Work out the finished part from the listing and answer in its coordinate system (mm). A direction names the side the tool comes from. Round coordinates to 2 decimals unless told otherwise and drop trailing zeros. Write each loop counter-clockwise with the first axis right and the second up, starting at its lowest first coordinate (ties: lowest second). Pieces come first, ordered by that corner, then holes. Notation, with made-up numbers: (17.5, 66.5) -> (74.5, 66.5) arc R10 cw to (74.5, 82.5) -> close; hole circle Ø11 at (17.25, 30.5). An arc over 180 degrees is marked (long way). One line per item, written item: value.
```python
from build123d import *

# Parameters (mm, degrees)
BOSS_EXTRUDE1_DEPTH  = 9.5
BOSS_EXTRUDE2_DEPTH  = 22
BOSS_EXTRUDE3_DEPTH  = 7.9
SKETCH5_R            = 11
SKETCH5_R_2          = 5
BOSS_EXTRUDE4_DEPTH  = 2
CUT_EXTRUDE1_START   = -3
SKETCH6_R            = 5
CUT_EXTRUDE1_DEPTH   = 3
SKETCH7_R            = 2.5
BOSS_EXTRUDE5_DEPTH  = 5
SKETCH8_R            = 2.5
BOSS_EXTRUDE6_DEPTH  = 22
CUT_EXTRUDE2_DEPTH   = 17
SKETCH11_W           = 3.2
SKETCH11_H           = 16
BOSS_EXTRUDE8_DEPTH  = 3.9
BOSS_EXTRUDE9_DEPTH  = 5.6
SKETCH13_W           = 0.930512921
SKETCH13_H           = 15
BOSS_EXTRUDE10_DEPTH = 3.9
SKETCH14_W           = 0.930512921
SKETCH14_H           = 15
BOSS_EXTRUDE11_DEPTH = 0.1
BOSS_EXTRUDE12_DEPTH = 5
SKETCH16_R           = 0.25
BOSS_EXTRUDE13_DEPTH = 5
SKETCH17_R           = 1.5
CUT_EXTRUDE3_DEPTH   = 5.5
SKETCH18_R           = 3.25
CUT_EXTRUDE4_DEPTH   = 3
CUT_EXTRUDE5_START   = -4
SKETCH20_R           = 1.5
CUT_EXTRUDE5_DEPTH   = 4
SKETCH21_R           = 4.5
CUT_EXTRUDE6_DEPTH   = 4


with BuildPart() as part:
    # Sketch1 → Boss-Extrude1 (new body)
    with BuildSketch(Plane.XY):
        Polygon((-17, 21), (-21, 17), (-21, -17), (-17, -21), (17, -21), (21, -17), (21, 17), (17, 21), align=None)
    extrude(amount=BOSS_EXTRUDE1_DEPTH)

    # Sketch2 → Boss-Extrude2 (add)
    with BuildSketch(Plane.XY.offset(9.5)):
        Polygon((14, 21.15), (21.15, 14), (21.15, -14), (14, -21.15), (-14, -21.15), (-21.15, -14), (-21.15, 14), (-14, 21.15), align=None)
    extrude(amount=BOSS_EXTRUDE2_DEPTH)

    # Sketch3 → Boss-Extrude3 (add)
    with BuildSketch(Plane.XY.offset(31.5)):
        Polygon((-17, 21), (17, 21), (21, 17), (21, -17), (17, -21), (-17, -21), (-21, -17), (-21, 17), align=None)
    extrude(amount=BOSS_EXTRUDE3_DEPTH)

    # Sketch5 → Boss-Extrude4 (add)
    with BuildSketch(Plane.XY.offset(39.4)):
        with Locations(Location((0, 0, 0), (0, 0, 180))):
            Circle(SKETCH5_R)
        Circle(SKETCH5_R_2, mode=Mode.SUBTRACT)
    extrude(amount=BOSS_EXTRUDE4_DEPTH)

    # Sketch6 → Cut-Extrude1 (cut)
    with BuildSketch(Plane.XY.offset(39.4).offset(CUT_EXTRUDE1_START)):
        Circle(SKETCH6_R)
    extrude(amount=CUT_EXTRUDE1_DEPTH, mode=Mode.SUBTRACT)

    # Sketch7 → Boss-Extrude5 (add)
    with BuildSketch(Plane.XY.offset(36.4)):
        with Locations(Location((0, 0, 0), (0, 0, 180))):
            Circle(SKETCH7_R)
    extrude(amount=BOSS_EXTRUDE5_DEPTH)

    # Sketch8 → Boss-Extrude6 (add)
    with BuildSketch(Plane.XY.offset(41.4)):
        with Locations(Location((0, 0, 0), (0, 0, 180))):
            Circle(SKETCH8_R)
    extrude(amount=BOSS_EXTRUDE6_DEPTH)

    # Sketch9 → Cut-Extrude2 (cut)
    with BuildSketch(Plane.XY.offset(63.4)):
        Polygon((-2.316645086, 2.1), (3.697939095, 2.1), (-0.123554347, 3.991048302), align=None)
    extrude(amount=-CUT_EXTRUDE2_DEPTH, mode=Mode.SUBTRACT)

    # Sketch11 → Boss-Extrude8 (add)
    with BuildSketch(Plane(origin=(21, 0, 0), x_dir=(0, 0, -1), z_dir=(1, 0, 0))):
        with Locations((-1.645589959, 0)):
            Rectangle(SKETCH11_W, SKETCH11_H)
    extrude(amount=BOSS_EXTRUDE8_DEPTH)

    # Sketch12 → Boss-Extrude9 (add)
    with BuildSketch(Plane(origin=(21, 0, 0), x_dir=(0, 0, -1), z_dir=(1, 0, 0))):
        Polygon((-9.5, 7.2), (-4.97610288, 7.2), (-4.97610288, -7.2), (-9.5, -7.2), (-9.5, -8), (-4.17610288, -8), (-4.17610288, -7.2), (-4.17610288, 7.2), (-4.17610288, 8), (-9.5, 8), align=None)
    extrude(amount=BOSS_EXTRUDE9_DEPTH)

    # Sketch13 → Boss-Extrude10 (add)
    with BuildSketch(Plane(origin=(21, 0, 0), x_dir=(0, 0, -1), z_dir=(1, 0, 0))):
        with Locations((-3.71084642, 0)):
            Rectangle(SKETCH13_W, SKETCH13_H)
    extrude(amount=BOSS_EXTRUDE10_DEPTH)

    # Sketch14 → Boss-Extrude11 (add)
    with BuildSketch(Plane(origin=(24.9, 0, 0), x_dir=(0, 0, -1), z_dir=(1, 0, 0))):
        with Locations((-3.71084642, 0)):
            Rectangle(SKETCH14_W, SKETCH14_H)
    extrude(amount=BOSS_EXTRUDE11_DEPTH)

    # Sketch15 → Boss-Extrude12 (add)
    with BuildSketch(Plane(origin=(21, 0, 0), x_dir=(0, 0, -1), z_dir=(1, 0, 0))):
        Polygon((-5.97610288, 6.2), (-9, 6.2), (-9, 4), (-9.5, 4), (-9.5, 6.7), (-9, 6.7), (-5.47610288, 6.7), (-5.47610288, -6.7), (-9, -6.7), (-9.5, -6.7), (-9.5, -4), (-9, -4), (-9, -6.2), (-5.97610288, -6.2), align=None)
    extrude(amount=BOSS_EXTRUDE12_DEPTH)

    # Sketch16 → Boss-Extrude13 (add)
    with BuildSketch(Plane(origin=(21, 0, 0), x_dir=(0, 0, -1), z_dir=(1, 0, 0))):
        with Locations(Location((-7.48805144, 5, 0), (0, 0, 270))):
            Circle(SKETCH16_R)
        with Locations(Location((-7.48805144, 3, 0), (0, 0, 270))):
            Circle(SKETCH16_R)
        with Locations(Location((-7.48805144, 1, 0), (0, 0, 270))):
            Circle(SKETCH16_R)
        with Locations(Location((-7.48805144, -1, 0), (0, 0, 270))):
            Circle(SKETCH16_R)
        with Locations(Location((-7.48805144, -3, 0), (0, 0, 270))):
            Circle(SKETCH16_R)
        with Locations(Location((-7.48805144, -5, 0), (0, 0, 270))):
            Circle(SKETCH16_R)
    extrude(amount=BOSS_EXTRUDE13_DEPTH)

    # Sketch17 → Cut-Extrude3 (cut)
    with BuildSketch(Plane.XY.offset(39.4)):
        with Locations((-15.5, 15.5)):
            Circle(SKETCH17_R)
        with Locations((15.5, 15.5)):
            Circle(SKETCH17_R)
        with Locations((15.5, -15.5)):
            Circle(SKETCH17_R)
        with Locations((-15.5, -15.5)):
            Circle(SKETCH17_R)
    extrude(amount=-CUT_EXTRUDE3_DEPTH, mode=Mode.SUBTRACT)

    # Sketch18 → Cut-Extrude4 (cut)
    with BuildSketch(Plane(origin=(0, 0, 0), x_dir=(-1, 0, 0), z_dir=(0, 0, -1))):
        with Locations((-15.5, 15.5)):
            Circle(SKETCH18_R)
        with Locations((15.5, 15.5)):
            Circle(SKETCH18_R)
        with Locations((15.5, -15.5)):
            Circle(SKETCH18_R)
        with Locations((-15.5, -15.5)):
            Circle(SKETCH18_R)
    extrude(amount=-CUT_EXTRUDE4_DEPTH, mode=Mode.SUBTRACT)

    # Sketch20 → Cut-Extrude5 (cut)
    with BuildSketch(Plane(origin=(0, 0, 3), x_dir=(-1, 0, 0), z_dir=(0, 0, -1)).offset(CUT_EXTRUDE5_START)):
        with Locations(Location((-15.5, 15.5, 0), (0, 0, 180))):
            Circle(SKETCH20_R)
        with Locations(Location((15.5, 15.5, 0), (0, 0, 180))):
            Circle(SKETCH20_R)
        with Locations(Location((-15.5, -15.5, 0), (0, 0, 180))):
            Circle(SKETCH20_R)
        with Locations(Location((15.5, -15.5, 0), (0, 0, 180))):
            Circle(SKETCH20_R)
    extrude(amount=CUT_EXTRUDE5_DEPTH, mode=Mode.SUBTRACT)

    # Sketch21 → Cut-Extrude6 (cut)
    with BuildSketch(Plane(origin=(0, 0, 0), x_dir=(-1, 0, 0), z_dir=(0, 0, -1))):
        Circle(SKETCH21_R)
    extrude(amount=-CUT_EXTRUDE6_DEPTH, mode=Mode.SUBTRACT)


solid = part.part
```
(1) Find section C-C on z = 18.5. Give the vertices of the cut face in (x, y), plus the area to 3 significant figures.
Reported:
outline: (-21.15, -14) -> (-14, -21.15) -> (14, -21.15) -> (21.15, -14) -> (21.15, 14) -> (14, 21.15) -> (-14, 21.15) -> (-21.15, 14) -> close
area: 1,690 mm2
(2) Find section D-D on x = 10. Give the vertices of the cut face in (y, z).
Reported:
outline: (-21.15, 9.5) -> (-21, 9.5) -> (-21, 0) -> (21, 0) -> (21, 9.5) -> (21.15, 9.5) -> (21.15, 31.5) -> (21, 31.5) -> (21, 39.4) -> (4.58, 39.4) -> (4.58, 41.4) -> (-4.58, 41.4) -> (-4.58, 39.4) -> (-21, 39.4) -> (-21, 31.5) -> (-21.15, 31.5) -> close
(3) Flat-ended cylindrical pins translate along their axes: pin 1 Ø3 at (x, y) = (-15, -14.5) entering from -Z; pin 2 Ø10 at (y, z) = (5, 32.5) entering from -X; pin 3 Ø3 at (y, z) = (0, 7.5) entering from +X; pin 4 Ø2.5 at (x, z) = (24.5, 7) entering from -Y. Find the tip coordinate at first contact, or state that the pin passes through.
Reported:
pin 1: stops at z = 3
pin 2: stops at x = -21.15
pin 3: stops at x = 26
pin 4: stops at y = -8
(4) A tool of negligible diameter and unlimited length cuts with its end or side. For faces 5 (the face through (24.9, 0, 2)), 6 (the face through (23, 6.2, 7)), 7 (the face through (-16, 16, 33.9)), 8 (the face through (0.59, 4.46, 1.97)), 9 (the face through (24, -5, 9.5)), from which of +Z, -Z, +X, -X, +Y, -Y can it reach the whole face along a straight path? Write none if from no direction.
Reported:
face 5: -Z, +X, +Y, -Y
face 6: +X
face 7: +Z
face 8: -Z
face 9: +Z, +X, +Y, -Y
(5) Find section A-A on z = 35. Give the vertices of the cut face in (x, y).
Reported:
outline: (-21, -17) -> (-17, -21) -> (17, -21) -> (21, -17) -> (21, 17) -> (17, 21) -> (-17, 21) -> (-21, 17) -> close; hole circle Ø3 at (-15.5, -15.5); hole circle Ø3 at (-15.5, 15.5); hole circle Ø3 at (15.5, -15.5); hole circle Ø3 at (15.5, 15.5)
(6) For a pull along Y with two mould halves and no side action, classify faces 1 (the face through (19, -19, 5)), 2 (the face through (23, 0, 5.476)), 3 (the face through (23, -5, 9)), 4 (the face through (19, 19, 5)) as pulls with the +Y half, pulls with the -Y half, needs draft (parallel to the pull), parting line crosses it, or undercut.
Reported:
face 1: pulls with the -Y half
face 2: undercut
face 3: undercut
face 4: pulls with the +Y half
(7) Find section B-B on x = 22.5. Give the number of separate pieces and of enclosed holes in the cut face, plus the area to 3 significant figures.
Reported:
separate pieces: 8
enclosed holes: 0
area: 98.8 mm2
(8) Consider probe 1 along X at (y, z) = (15.5, 5.2); probe 2 along Z at (x, y) = (22, -5.5). Determine where each line is inside the solid, lowest interval first.
Reported:
probe 1: x = -21 to -17, -14 to 14, 17 to 21
probe 2: z = 0.05 to 4.98, 5.48 to 5.98, 9 to 9.5
